For this review, take the finished solid that the model builds, in its own axes (mm). Coordinates: 2 decimals unless noted, no trailing zeros. Order: outer loops, then holes, each group sorted by start corner. A loop starts at its lowest first (then second) coordinate and runs counter-clockwise, first axis right, second up.
from build123d import *

# Parameters (mm, degrees)
SKETCH1_R           = 7
BOSS_EXTRUDE1_DEPTH = 10
SHELL1_T            = -1
SKETCH2_R           = 1.5
CUT_EXTRUDE1_DEPTH  = 10


with BuildPart() as part:
    # Sketch1 → Boss-Extrude1 (new body)
    with BuildSketch(Plane(origin=(0, 0, 0), x_dir=(1, 0, 0), z_dir=(0, 1, 0))):
        with Locations(Location((0, 0, 0), (0, 0, 270))):
            Circle(SKETCH1_R)
    extrude(amount=BOSS_EXTRUDE1_DEPTH)

    # Shell1
    shell1_openings = [part.faces().sort_by_distance(p)[0] for p in [
        (0, 0, 0),
    ]]
    offset(amount=SHELL1_T, openings=shell1_openings, kind=Kind.INTERSECTION)

    # Sketch2 → Cut-Extrude1 (cut)
    with BuildSketch(Plane(origin=(0, 9, 0), x_dir=(-1, 0, 0), z_dir=(0, -1, 0))):
        with Locations(Location((0, 0, 0), (0, 0, 90))):
            Circle(SKETCH2_R)
    extrude(amount=-CUT_EXTRUDE1_DEPTH, mode=Mode.SUBTRACT)


solid = part.part
1. Take a section at D-D, the plane x = 1.75. Give the boundary of the cut face in (y, z).
Answer below:
outline: (0, -6.78) - (10, -6.78) - (10, 6.78) - (0, 6.78) - (0, 5.74) - (9, 5.74) - (9, -5.74) - (0, -5.74) - close
2. The part is to be moulded in two halves that separate along X. For faces 1 (the face through (1.802, 4.437, 5.723)), 2 (the face through (-1.2, 9, 1.2)), 3 (the face through (-6.834, 4.93, -1.517)), 4 (the face through (2, 10, 0)), say which applies: +X half, -X half, draft (parallel to the pull), parting line (faces both ways), or undercut.
Answer below:
face 1: undercut
face 2: undercut
face 3: parting line
face 4: draft
3. Take a section at A-A, the plane z = 0. Give the boundary of the cut face in (x, y), plus the area to 3 significant figures.
Answer below:
outline: (-7, 0) - (-6, 0) - (-6, 9) - (-1.5, 9) - (-1.5, 10) - (-7, 10) - close; (1.5, 9) - (6, 9) - (6, 0) - (7, 0) - (7, 10) - (1.5, 10) - close
area: 29.0 mm2
4. Take a section at B-B, the plane x = 0. Give the boundary of the cut face in (y, z), plus the area to 3 significant figures.
Answer below:
outline: (0, -7) - (10, -7) - (10, -1.5) - (9, -1.5) - (9, -6) - (0, -6) - close; (0, 6) - (9, 6) - (9, 1.5) - (10, 1.5) - (10, 7) - (0, 7) - close
area: 29.0 mm2
5. To check wall thickness, follow L1, parallel to X at y = 9.5, z = 0; L2, parallel to X at y = 5.5, z = 0; L3, parallel to Y at x = -2.5, z = 1. State the ranges of each line that lie inside material, in increasing order.
Answer below:
L1: x = -7 to -1.5, 1.5 to 7
L2: x = -7 to -6, 6 to 7
L3: y = 9 to 10
6. Clearance check with flat-ended pins moving along their axes: pin 1 Ø1 at (y, z) = (3, 2.5) entering from +X; pin 2 Ø2.5 at (x, z) = (0, 0) entering from -Y. State where each tip first meets the part, or that it passes through.
Answer below:
pin 1: stops at x = 6.71
pin 2: passes through
7. Take a section at C-C, the plane y = 2. Give the boundary of the cut face in (x, z), plus the area to 3 significant figures.
Answer below:
outline: circle Ø14 at (0, 0); hole circle Ø12 at (0, 0)
area: 40.8 mm2
